Model file for the job. Use its own axes, mm. Round coordinates to 2 decimals unless told otherwise and drop trailing zeros. Loops run counter-clockwise (first coordinate to the right, second up) from the corner with the lowest first, then second, coordinate; pieces in that order, holes last. Notation, with made-up numbers: M 24.5,49 L 30.5,49 A37 cw 30.5,86 Z; hole C -11.75,15 d1. An arc over 180 degrees is marked long. Use a Markdown table: item, result. Add a question column.
Q1. Cut at A-A (z = 0.4). State how many separate pieces and enclosed holes the cut face has, plus the area to 3 significant figures.
Q2. Pin check, flat tips, straight feed: pin 1 (0.6 mm diameter, centred on x = -37, z = 1, fed in from +Y); pin 2 (0.9 mm diameter, centred on x = -19, z = 1, fed in from +Y); pin 3 (0.6 mm diameter, centred on x = -1.5, z = 1, fed in from +Y). Stop position of each tip, or through.
Q3. Cut at C-C (y = 0.5). Give the cut face in (x, z), plus the area to 3 significant figures.
Q4. Probe line 1 (Y direction, x = -23, z = 0.5); line 2 (X direction, y = -9, z = 1.1); line 3 (Y direction, x = 31.5, z = 1.35). List the from-to ranges inside material, lowest first. Write a range as from..to.
Q5. Cut at B-B (x = 37.5). Give the cut face in (y, z).
from build123d import *

# Parameters (mm, degrees)
F2_DEPTH = 2
F3_W     = 0.40073
F3_H     = 3.094508
F3_W_2   = 0.445254
F3_H_2   = 4.318954
F3_H_3   = 5.565662
F3_H_4   = 6.723319
F3_W_3   = 0.445252
F3_H_5   = 7.725138
F3_H_6   = 8.370755
F3_H_7   = 8.83827
F3_H_8   = 9.105423
F3_W_4   = 0.445253
F3_H_9   = 9.506151
F3_H_10  = 9.439363
F3_H_11  = 9.083159
F3_H_12  = 8.459806
F3_W_5   = 0.448172
F3_H_13  = 8.174662
F3_H_14  = 6.776365
F3_H_15  = 5.736604
F3_H_16  = 4.678918
F3_W_6   = 0.451199
F3_H_17  = 3.560012
F4_DEPTH = 2


with BuildPart() as f2:
    # F1 (on face) → F2 (new body)
    with BuildSketch(Plane.XY):
        Polygon((-42.565533, -25.966065), (-42.565533, -27.660457), (0, -27.660457), (0, -25.966065), (-3.254796, -25.966065), (-4.865278, -25.966065), (-6.80548, -25.966065), (-7.284604, -25.966065), (-8.611036, -25.966065), (-9.190797, -25.966065), (-10.747001, -25.966065), (-11.576914, -25.966065), (-13.527635, -25.966065), (-14.543153, -25.966065), (-16.00546, -25.966065), (-17.032834, -25.966065), (-18.660922, -25.966065), (-19.680227, -25.966065), (-21.282767, -25.966065), (-22.327718, -25.966065), (-24.128009, -25.966065), (-24.945042, -25.966065), (-26.6696, -25.966065), (-27.674529, -25.966065), (-29.783733, -25.966065), (-30.905583, -25.966065), (-33.341274, -25.966065), (-34.150291, -25.966065), (-36.62416, -25.966065), (-37.416613, -25.966065), (-39.790157, -25.966065), (-41.272748, -25.966065), align=None)
        Polygon((0, -25.966065), (0, -27.660457), (0, -29.807076), (42.442255, -29.978171), (42.442255, -25.966065), (37.837461, -25.966065), (35.959285, -25.966065), (35.959285, -19.634349), (31.794641, -12.611612), (22.485428, -12.611612), (22.485428, -3.422375), (24.526922, -3.422375), (20.198954, 5.84349), (16.263861, -3.422375), (18.525192, -3.422375), (18.525192, -19.802407), (14.995469, -16.15097), (11.306624, -19.716855), (11.306624, -25.966065), (9.322134, -25.966065), (9.322134, -20.964459), (6.251046, -17.787471), (2.015062, -20.964459), (2.015062, -25.966065), align=None)
        with BuildLine():
            ThreePointArc((-3.254796, -25.966065), (-22.263772, -15.386694), (-41.272748, -25.966065))
            Line((-41.272748, -25.966065), (-39.790157, -25.966065))
            ThreePointArc((-39.790157, -25.966065), (-38.665481, -24.491199), (-37.416613, -23.119903))
            ThreePointArc((-37.416613, -23.119903), (-37.025265, -22.73615), (-36.62416, -22.362606))
            ThreePointArc((-36.62416, -22.362606), (-35.422916, -21.350754), (-34.150291, -20.430287))
            ThreePointArc((-34.150291, -20.430287), (-33.748684, -20.16832), (-33.341274, -19.915471))
            ThreePointArc((-33.341274, -19.915471), (-32.143886, -19.242725), (-30.905583, -18.648645))
            ThreePointArc((-30.905583, -18.648645), (-30.347908, -18.41234), (-29.783733, -18.192007))
            ThreePointArc((-29.783733, -18.192007), (-28.7378, -17.831313), (-27.674529, -17.525486))
            ThreePointArc((-27.674529, -17.525486), (-27.17349, -17.401847), (-26.6696, -17.290397))
            ThreePointArc((-26.6696, -17.290397), (-25.810262, -17.129587), (-24.945042, -17.00422))
            ThreePointArc((-24.945042, -17.00422), (-24.536938, -16.957621), (-24.128009, -16.91891))
            ThreePointArc((-24.128009, -16.91891), (-23.228672, -16.861684), (-22.327718, -16.842597))
            ThreePointArc((-22.327718, -16.842597), (-21.805084, -16.849018), (-21.282767, -16.868277))
            ThreePointArc((-21.282767, -16.868277), (-20.480176, -16.922976), (-19.680227, -17.007981))
            ThreePointArc((-19.680227, -17.007981), (-19.169648, -17.078313), (-18.660922, -17.160994))
            ThreePointArc((-18.660922, -17.160994), (-17.843441, -17.320594), (-17.032834, -17.512072))
            ThreePointArc((-17.032834, -17.512072), (-16.517316, -17.651472), (-16.00546, -17.803769))
            ThreePointArc((-16.00546, -17.803769), (-15.269621, -18.047594), (-14.543153, -18.318065))
            ThreePointArc((-14.543153, -18.318065), (-14.032607, -18.526492), (-13.527635, -18.748083))
            ThreePointArc((-13.527635, -18.748083), (-12.539214, -19.228362), (-11.576914, -19.759042))
            ThreePointArc((-11.576914, -19.759042), (-11.159024, -20.010256), (-10.747001, -20.270981))
            ThreePointArc((-10.747001, -20.270981), (-9.956389, -20.809703), (-9.190797, -21.383427))
            ThreePointArc((-9.190797, -21.383427), (-8.602301, -21.862673), (-8.031275, -22.362606))
            ThreePointArc((-8.031275, -22.362606), (-7.653628, -22.713766), (-7.284604, -23.073977))
            ThreePointArc((-7.284604, -23.073977), (-7.043039, -23.319504), (-6.80548, -23.568909))
            ThreePointArc((-6.80548, -23.568909), (-5.791883, -24.732282), (-4.865278, -25.966065))
            Line((-4.865278, -25.966065), (-3.254796, -25.966065))
        make_face()
    extrude(amount=F2_DEPTH)

    # F3 (on face) → F4 (join)
    with BuildSketch(Plane.XY):
        with Locations((-37.955668, -24.606134)):
            Rectangle(F3_W, F3_H)
        with Locations((-36.330495, -23.904861)):
            Rectangle(F3_W_2, F3_H_2)
        with Locations((-34.772109, -23.236981)):
            Rectangle(F3_W_2, F3_H_3)
        with Locations((-32.879785, -22.658152)):
            Rectangle(F3_W_2, F3_H_4)
        with Locations((-31.388187, -22.201769)):
            Rectangle(F3_W_3, F3_H_5)
        with Locations((-29.696227, -21.87896)):
            Rectangle(F3_W_3, F3_H_6)
        with Locations((-27.915214, -21.689728)):
            Rectangle(F3_W_3, F3_H_7)
        with Locations((-26.401355, -21.533888)):
            Rectangle(F3_W_3, F3_H_8)
        with Locations((-24.798444, -21.333524)):
            Rectangle(F3_W_4, F3_H_9)
        with Locations((-23.373634, -21.333524)):
            Rectangle(F3_W_4, F3_H_9)
        with Locations((-22.037876, -21.30013)):
            Rectangle(F3_W_3, F3_H_10)
        with Locations((-20.702117, -21.333524)):
            Rectangle(F3_W_3, F3_H_9)
        with Locations((-19.321834, -21.30013)):
            Rectangle(F3_W_3, F3_H_10)
        with Locations((-17.763448, -21.30013)):
            Rectangle(F3_W_3, F3_H_10)
        with Locations((-16.249589, -21.567283)):
            Rectangle(F3_W_3, F3_H_11)
        with Locations((-14.646677, -21.834435)):
            Rectangle(F3_W_3, F3_H_12)
        with Locations((-13.227864, -21.954445)):
            Rectangle(F3_W_5, F3_H_13)
        with Locations((-11.722005, -22.653593)):
            Rectangle(F3_W_5, F3_H_14)
        with Locations((-10.216147, -23.24518)):
            Rectangle(F3_W_5, F3_H_15)
        with Locations((-8.477238, -23.720243)):
            Rectangle(F3_W_5, F3_H_16)
        with Locations((-6.799724, -24.328857)):
            Rectangle(F3_W_6, F3_H_17)
    extrude(amount=F4_DEPTH)


solid = f2.part
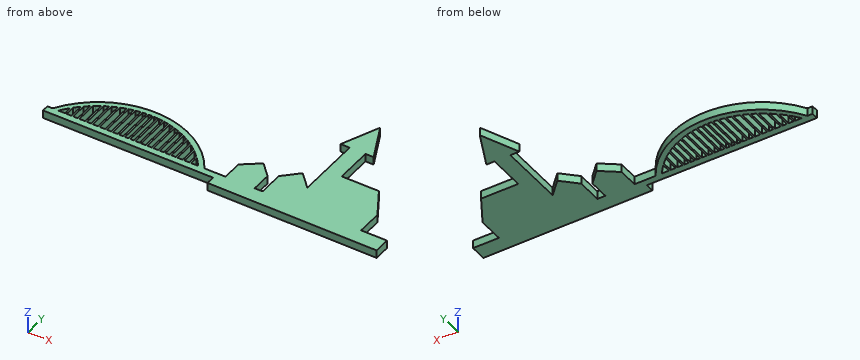
Checked values:
| question | item | result |
|---|---|---|
| 1 | separate pieces | 1 |
| 1 | enclosed holes | 22 |
| 1 | area | 762 mm^2 |
| 2 | pin 1 | stops at y = -20.67 |
| 2 | pin 2 | stops at y = -15.56 |
| 2 | pin 3 | stops at y = -25.97 |
| 3 | outline | M 17.93,0 L 22.69,0 L 22.69,2 L 17.93,2 Z |
| 3 | area | 9.53 mm^2 |
| 4 | line 1 | y = -27.66..-25.97, -16.85..-15.4 |
| 4 | line 2 | x = 18.53..22.49 |
| 4 | line 3 | y = -29.93..-12.61 |
| 5 | outline | M -29.96,0 L -25.97,0 L -25.97,2 L -29.96,2 Z |
